For this review, take the finished solid that the model builds, in its own axes (mm). Face numbers are marked on the shaded views. Round coordinates to 2 decimals unless told otherwise and drop trailing zeros. Write each loop counter-clockwise with the first axis right and the second up, starting at its lowest first coordinate (ties: lowest second). Pieces come first, ordered by that corner, then holes.
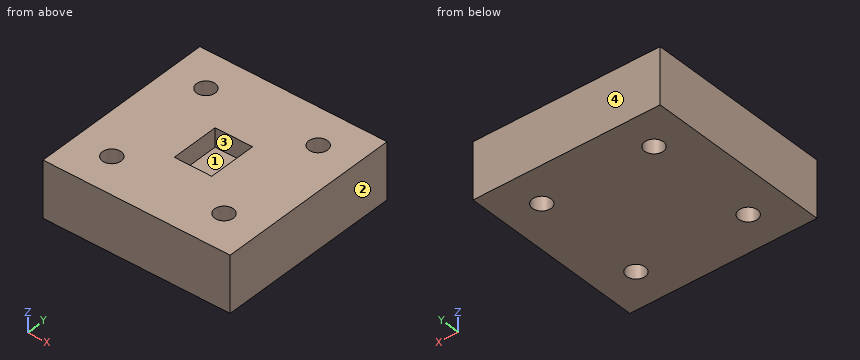
Autodesk Fusion 360 part; units mm, degrees
sketch "Esquisse1" plane through (0, 0, 0) normal (0, 0, 1) x (1, 0, 0)
  line L0 (0, 0) -> (50, 0)
  line L1 (50, 0) -> (50, 50)
  line L2 (50, 50) -> (0, 50)
  line L3 (0, 50) -> (0, 0)
  circle A0 centre (10, 40) radius 2.5
  circle A1 centre (40, 40) radius 2.5
  circle A2 centre (10, 10) radius 2.5
  circle A3 centre (40, 10) radius 2.5
  dimension "d1" = 5
  dimension "d2" = 5
  dimension "d3" = 5
  dimension "d4" = 5
extrude "Extrusion1" add sketch "Esquisse1" along normal blind 15
sketch "Esquisse2" plane through (0, 0, 15) normal (0, 0, 1) x (-1, 0, 0)
  circle A0 centre (-10, -40) radius 2.5
  circle A1 centre (-10, -10) radius 2.5
  circle A2 centre (-40, -10) radius 2.5
  circle A3 centre (-40, -40) radius 2.5
  line L0 (0, -50) -> (0, 0)
  line L1 (0, 0) -> (-50, 0)
  line L2 (-50, 0) -> (-50, -50)
  line L3 (-50, -50) -> (0, -50)
  line L4 (0, -25) -> (-20, -25)
  line L5 (-20, -25) -> (-30, -25)
  line L6 (-30, -25) -> (-30, -30)
  line L7 (-30, -30) -> (-20, -30)
  line L8 (-20, -30) -> (-20, -20)
  line L9 (-20, -20) -> (-30, -20)
  line L10 (-30, -20) -> (-30, -25)
  line L11 (-30, -20) -> (-30, -18)
  line L12 (-30, -18) -> (-20, -18)
  line L13 (-20, -18) -> (-20, -20)
  line L14 (-30, -30) -> (-30, -31)
  line L15 (-30, -31) -> (-20, -31)
  line L16 (-20, -31) -> (-20, -30)
  dimension "d7" = 2
  dimension "d8" = 1
extrude "Extrusion2" cut sketch "Esquisse2" against normal blind 5 contours L5 L6 L7 L8 | L5 L8 L9 L10 | L7 L14 L15 L16 | L9 L11 L12 L13
(1) We need section C-C, the plane z = 7.25. Give the boundary of the cut face in (x, y).
Geometry check:
outline: (0, 0) - (50, 0) - (50, 50) - (0, 50) - close; hole circle Ø5 at (10, 10); hole circle Ø5 at (10, 40); hole circle Ø5 at (40, 10); hole circle Ø5 at (40, 40)
(2) For pin 1 Ø3 at (x, y) = (40, 10) entering from +Z; pin 2 Ø5 at (x, y) = (25, 25.5) entering from +Z, all flat-tipped, find the tip position at first contact; note any pin that passes through.
Geometry check:
pin 1: passes through
pin 2: stops at z = 10
(3) For line 1 along Y through (x, z) = (10, 4.25); line 2 along X through (y, z) = (39.5, 4.25); line 3 along X through (y, z) = (25, 14), list the stretches that pass through material, from the lowest coordinate up.
Geometry check:
line 1: y = 0 to 7.5, 12.5 to 37.5, 42.5 to 50
line 2: x = 0 to 7.55, 12.45 to 37.55, 42.45 to 50
line 3: x = 0 to 20, 30 to 50
(4) Mouldability with a two-part tool opening along X and no side actions: class the marked faces 1, 2, 3 and 4 as pulls with the +X half, pulls with the -X half, needs draft (parallel to the pull), parting line crosses it, or undercut.
Geometry check:
face 1: undercut
face 2: pulls with the +X half
face 3: undercut
face 4: needs draft
(5) We need section A-A, the plane x = 10. Give the boundary of the cut face in (y, z), and give its area (3 significant figures).
Geometry check:
outline: (0, 0) - (7.5, 0) - (7.5, 15) - (0, 15) - close; (12.5, 0) - (37.5, 0) - (37.5, 15) - (12.5, 15) - close; (42.5, 0) - (50, 0) - (50, 15) - (42.5, 15) - close
area: 600 mm2
(6) We need section D-D, the plane y = 19.5. Give the boundary of the cut face in (x, z).
Geometry check:
outline: (0, 0) - (50, 0) - (50, 15) - (30, 15) - (30, 10) - (20, 10) - (20, 15) - (0, 15) - close
